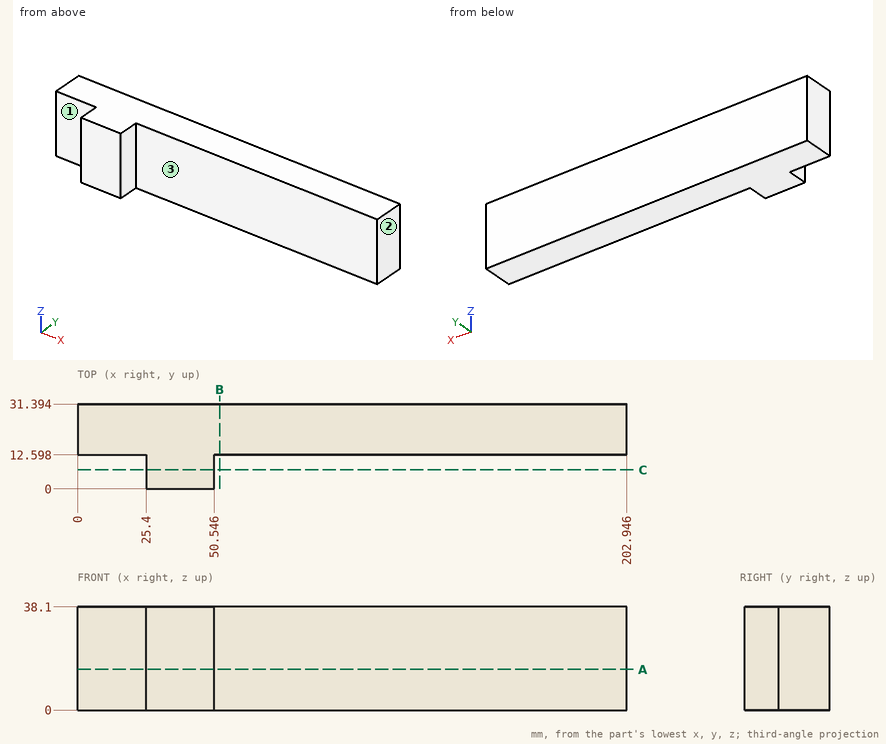
Source: three-view drawing plus pictorial views. Frame: mm from the lowest corner of the part. A direction names the side the tool comes from. Give positions to 0.01 mm unless a question says otherwise; leave off trailing zeros. Order: outer loops, then holes, each group sorted by start corner. A loop starts at its lowest first (then second) coordinate and runs counter-clockwise, first axis right, second up. Notation, with made-up numbers: (31, 28.5) - (46, 28.5) arc R26 ccw to (46, 63.5) - close; hole circle Ø3 at (54.5, 0). An arc over 180 degrees is marked (long way). Answer as a JSON object with one key per item and string values. Group by question number.
Q1. First-contact query: pin 1 Ø4 at (y, z) = (3.5, 13.5) entering from -X; pin 2 Ø14 at (y, z) = (3.5, 17) entering from +X; pin 3 Ø11.5 at (x, z) = (133.5, 10.5) entering from -Y. Flat tips, straight axial feed; report the tip coordinate or a pass-through.
Q2. Set-up query: the marked faces 1, 2 and 3. Return all of +Z, -Z, +X, -X, +Y, -Y with unobstructed straight access to the full face (end or side cutting, diameter ignored); none if empty.
Q3. Cut plane A-A, the plane z = 15. Output: boundary loops of the cut face in (x, y) (1 decimal), then the cut area to 3 significant figures.
Q4. Cut plane B-B, the plane x = 52.5. Output: boundary loops of the cut face in (y, z) (1 decimal).
Q5. Cut plane C-C, the plane y = 7. Output: boundary loops of the cut face in (x, z).
Q6. Line query: probe 1 along Y at (x, z) = (163.5, 23.5) (1 decimal); probe 2 along X at (y, z) = (6, 18). Output: solid intervals per line, ascending.
Results:
{
 "1": {"pin 1": "x = 25.4", "pin 2": "x = 50.55", "pin 3": "y = 12.6"},
 "2": {"face 1": "+Z, -Z, -X, -Y", "face 2": "+Z, -Z, +X, +Y, -Y", "face 3": "+Z, -Z, +X, -Y"},
 "3": {"outline": "(0, 12.6) - (25.4, 12.6) - (25.4, 0) - (50.5, 0) - (50.5, 12.6) - (202.9, 12.6) - (202.9, 31.4) - (0, 31.4) - close", "area": "4,130 mm^2"},
 "4": {"outline": "(12.6, 0) - (31.4, 0) - (31.4, 38.1) - (12.6, 38.1) - close"},
 "5": {"outline": "(25.4, 0) - (50.55, 0) - (50.55, 38.1) - (25.4, 38.1) - close"},
 "6": {"probe 1": "12.6 to 31.4", "probe 2": "25.4 to 50.55"}
}
